from build123d import *

# Parameters (mm, degrees)
F0_R     = 9.525
F1_DEPTH = 44.45
F2_DEPTH = 44.45
F3_DEPTH = 44.45
F4_DEPTH = 44.45
F5_DEPTH = 44.45
F6_DEPTH = 44.45
F7_DEPTH = 44.45
F8_DEPTH = 25.4
F9_DEPTH = 19.05


with BuildPart() as f1:
    # F0 (on Top) → F1 (new body)
    with BuildSketch(Plane.XY):
        with BuildLine():
            Line((5.1747410867, 18.3336999726), (1.9060083062, 18.9544093112))
            ThreePointArc((1.9060083062, 18.9544093112), (0.0969078237, 19.0497535122), (-1.7130690518, 18.9728198859))
            Line((-1.7130690518, 18.9728198859), (-5.3677419125, 18.2781248152))
            ThreePointArc((-5.3677419125, 18.2781248152), (-19.05, 0), (-5.3677419125, -18.2781248152))
            Line((-5.3677419125, -18.2781248152), (-1.7130690518, -18.9728198859))
            ThreePointArc((-1.7130690518, -18.9728198859), (0.0969078237, -19.0497535122), (1.9060083062, -18.9544093112))
            Line((1.9060083062, -18.9544093112), (5.1747410867, -18.3336999726))
            ThreePointArc((5.1747410867, -18.3336999726), (15.1901500602, -11.4961663675), (19.05, 0))
            ThreePointArc((19.05, 0), (15.1901500602, 11.4961663675), (5.1747410867, 18.3336999726))
        make_face()
        Circle(F0_R, mode=Mode.SUBTRACT)
        with BuildLine():
            Line((51.6444474156, 9.5094299521), (5.1747410867, 18.3336999726))
            ThreePointArc((5.1747410867, 18.3336999726), (15.1901500602, 11.4961663675), (19.05, 0))
            ThreePointArc((19.05, 0), (15.1901500602, -11.4961663675), (5.1747410867, -18.3336999726))
            Line((5.1747410867, -18.3336999726), (51.6444474156, -9.5094299521))
            Line((51.6444474156, -9.5094299521), (101.722291385, 0))
            Line((101.722291385, 0), (51.6444474156, 9.5094299521))
        make_face()
    extrude(amount=F1_DEPTH)

    # F0 (on Top) → F2 (join)
    with BuildSketch(Plane.XY):
        with BuildLine():
            Line((0, 65.538806632), (1.9060083062, 18.9544093112))
            ThreePointArc((1.9060083062, 18.9544093112), (3.5539517459, 18.7155530773), (5.1747410867, 18.3336999726))
            Line((5.1747410867, 18.3336999726), (51.6444474156, 9.5094299521))
            Line((51.6444474156, 9.5094299521), (0, 65.538806632))
        make_face()
    extrude(amount=F2_DEPTH)

    # F0 (on Top) → F3 (join)
    with BuildSketch(Plane.XY):
        with BuildLine():
            ThreePointArc((-5.3677419125, -18.2781248152), (-19.05, 0), (-5.3677419125, 18.2781248152))
            Line((-5.3677419125, 18.2781248152), (-51.6194616924, 9.486409943))
            Line((-51.6194616924, 9.486409943), (-101.5258543329, 0))
            Line((-101.5258543329, 0), (-51.6194616924, -9.486409943))
            Line((-51.6194616924, -9.486409943), (-5.3677419125, -18.2781248152))
        make_face()
    extrude(amount=F3_DEPTH)

    # F0 (on Top) → F4 (join)
    with BuildSketch(Plane.XY):
        with BuildLine():
            ThreePointArc((1.9060083062, -18.9544093112), (0.0969078237, -19.0497535122), (-1.7130690518, -18.9728198859))
            Line((-1.7130690518, -18.9728198859), (0, -65.538806632))
            Line((0, -65.538806632), (1.9060083062, -18.9544093112))
        make_face()
    extrude(amount=F4_DEPTH)

    # F0 (on Top) → F5 (join)
    with BuildSketch(Plane.XY):
        with BuildLine():
            ThreePointArc((-1.7130690518, 18.9728198859), (0.0969078237, 19.0497535122), (1.9060083062, 18.9544093112))
            Line((1.9060083062, 18.9544093112), (0, 65.538806632))
            Line((0, 65.538806632), (-1.7130690518, 18.9728198859))
        make_face()
    extrude(amount=F5_DEPTH)

    # F0 (on Top) → F6 (join)
    with BuildSketch(Plane.XY):
        with BuildLine():
            ThreePointArc((-1.7130690518, -18.9728198859), (-3.5574037286, -18.7148972402), (-5.3677419125, -18.2781248152))
            Line((-5.3677419125, -18.2781248152), (-51.6194616924, -9.486409943))
            Line((-51.6194616924, -9.486409943), (0, -65.538806632))
            Line((0, -65.538806632), (-1.7130690518, -18.9728198859))
        make_face()
        with BuildLine():
            Line((51.6444474156, -9.5094299521), (5.1747410867, -18.3336999726))
            ThreePointArc((5.1747410867, -18.3336999726), (3.5539517459, -18.7155530773), (1.9060083062, -18.9544093112))
            Line((1.9060083062, -18.9544093112), (0, -65.538806632))
            Line((0, -65.538806632), (51.6444474156, -9.5094299521))
        make_face()
    extrude(amount=F6_DEPTH)

    # F0 (on Top) → F7 (join)
    with BuildSketch(Plane.XY):
        with BuildLine():
            Line((0, 65.538806632), (1.9060083062, 18.9544093112))
            ThreePointArc((1.9060083062, 18.9544093112), (3.5539517459, 18.7155530773), (5.1747410867, 18.3336999726))
            Line((5.1747410867, 18.3336999726), (51.6444474156, 9.5094299521))
            Line((51.6444474156, 9.5094299521), (0, 65.538806632))
        make_face()
    extrude(amount=F7_DEPTH)

    # F0 (on Top) → F8 (join)
    with BuildSketch(Plane.XY):
        with BuildLine():
            ThreePointArc((-5.3677419125, 18.2781248152), (-3.5574037286, 18.7148972402), (-1.7130690518, 18.9728198859))
            Line((-1.7130690518, 18.9728198859), (0, 65.538806632))
            Line((0, 65.538806632), (-51.6194616924, 9.486409943))
            Line((-51.6194616924, 9.486409943), (-5.3677419125, 18.2781248152))
        make_face()
    extrude(amount=F8_DEPTH)

    # F9 (add): a face of the model
    f9_faces = [f1.faces().sort_by_distance(p)[0] for p in [
        (-17.7802963079, 31.335159678, 25.4),
    ]]
    extrude(f9_faces, amount=F9_DEPTH)


solid = f1.part
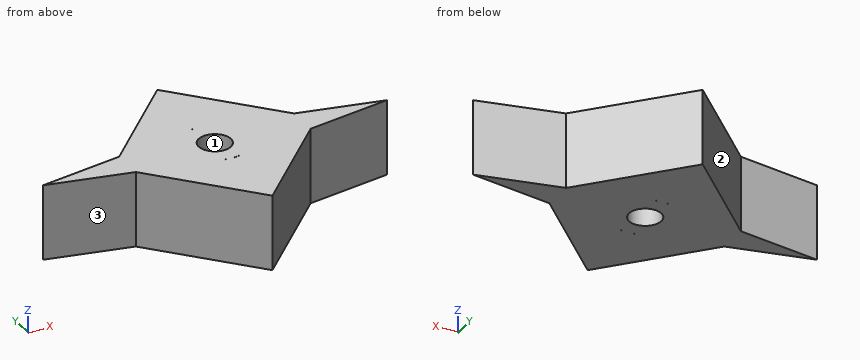
Verification items for the finished model (mm, model axes). Face numbers are marked on the shaded views. Round coordinates to 2 decimals unless told otherwise and drop trailing zeros. Write each loop counter-clockwise with the first axis right and the second up, starting at its lowest first coordinate (ties: lowest second). Pieces come first, ordered by that corner, then holes.
(1) Material ranges on line 1 (Y direction, x = 0, z = 26) (3 decimals); line 2 (Y direction, x = 72.5, z = 39.5); line 3 (X direction, y = 22, z = 38), recorded low to high.
Returned:
line 1: y = -65.539 to -9.525, 9.525 to 65.539
line 2: y = -5.55 to 5.55
line 3: x = -40.1 to 40.13
(2) Section check A-A (z = 39). Enter the section's corners in (x, y) (3 decimals), plus the area to 3 significant figures.
Returned:
outline: (-101.526, 0) - (-51.619, -9.486) - (0, -65.539) - (51.644, -9.509) - (101.722, 0) - (51.644, 9.509) - (0, 65.539) - (-51.619, 9.486) - close; hole circle Ø19.05 at (0, 0); hole (-5.368, -18.278) arc R19.05 ccw to (-1.713, -18.973) - close; hole (-5.368, 18.278) - (-1.713, 18.973) arc R19.05 ccw to start; hole (1.906, -18.954) arc R19.05 ccw to (5.175, -18.334) - close; hole (1.906, 18.954) - (5.175, 18.334) arc R19.05 ccw to start
area: 8,410 mm2
(3) Section check D-D (y = 29). Enter the section's corners in (x, z), plus the area to 3 significant figures.
Returned:
outline: (-33.65, 0) - (33.68, 0) - (33.68, 44.45) - (-33.65, 44.45) - close
area: 2,990 mm2
(4) Depth check by flat-ended pin: pin 1 Ø3 at (x, z) = (43.5, 19) entering from +Y; pin 2 Ø12 at (x, z) = (16.5, 38) entering from -Y; pin 3 Ø12 at (y, z) = (46, 36) entering from +X. Enter the tip coordinate at first touch or a pass-through.
Returned:
pin 1: stops at y = 19.97
pin 2: stops at y = -54.15
pin 3: stops at x = 23.54
(5) Mould release check, pull along Y, two halves, no side actions. Record for the marked faces 1, 2 and 3: pulls with the +Y half, pulls with the -Y half, needs draft (parallel to the pull), parting line crosses it, or undercut.
Returned:
face 1: undercut
face 2: pulls with the +Y half
face 3: pulls with the -Y half
(6) Section check C-C (x = 14). Enter the section's corners in (y, z), plus the area to 3 significant figures.
Returned:
outline: (-50.35, 0) - (50.35, 0) - (50.35, 44.45) - (-50.35, 44.45) - close
area: 4,480 mm2
(7) Section check B-B (y = 2). Enter the section's corners in (x, z).
Returned:
outline: (-91, 0) - (-9.31, 0) - (-9.31, 44.45) - (-91, 44.45) - close; (9.31, 0) - (91.19, 0) - (91.19, 44.45) - (9.31, 44.45) - close
